Can you work these out from the model? Positions are in its coordinate system, mm. Face numbers are marked on the shaded views. Round coordinates to 2 decimals unless told otherwise and drop trailing zeros. Loops run counter-clockwise (first coordinate to the right, second up) from the corner with the lowest first, then second, coordinate; pieces in that order, holes last. Notation, with made-up numbers: M 0,64.25 L 27,64.25 A20 ccw 27,81.25 Z; hole C -31,37 d2. An arc over 180 degrees is marked long. Return JSON: item names as keys, results as strings.
```python
from build123d import *

# Parameters (mm, degrees)
BOSS_EXTRUDE1_DEPTH = 56.3
SKETCH2_R           = 8.37
CUT_EXTRUDE1_DEPTH  = 109.485473941


with BuildPart() as part:
    # Sketch1 → Boss-Extrude1 (new body)
    with BuildSketch(Plane(origin=(0, 0, 0), x_dir=(1, 0, 0), z_dir=(0, 1, 0))):
        with BuildLine():
            Line((-85.3, 58.95), (-87.3, 58.95))
            Line((-87.3, 58.95), (-87.3, 65.95))
            Line((-87.3, 65.95), (-82, 65.95))
            Line((-82, 65.95), (-57.085698874, 65.95))
            ThreePointArc((-57.085698874, 65.95), (-30.460620038, 81.733286627), (0, 87.224878997))
            ThreePointArc((0, 87.224878997), (30.460620038, 81.733286627), (57.085698874, 65.95))
            Line((57.085698874, 65.95), (82, 65.95))
            Line((82, 65.95), (87.3, 65.95))
            Line((87.3, 65.95), (87.3, 58.95))
            Line((87.3, 58.95), (85.3, 58.95))
            Line((85.3, 58.95), (85.3, 63.95))
            Line((85.3, 63.95), (82.7, 63.95))
            Line((82.7, 63.95), (82.7, 55.95))
            Line((82.7, 55.95), (77.3, 55.95))
            Line((77.3, 55.95), (77.3, 58.692745098))
            Line((77.3, 58.692745098), (78.85, 58.692745098))
            Line((78.85, 58.692745098), (79.85, 57.359411765))
            Line((79.85, 57.359411765), (81.3, 57.359411765))
            Line((81.3, 57.359411765), (81.3, 63.95))
            Line((81.3, 63.95), (56.335401836, 63.95))
            ThreePointArc((56.335401836, 63.95), (30.109375518, 79.728950237), (0, 85.224878997))
            ThreePointArc((0, 85.224878997), (-30.109375518, 79.728950237), (-56.335401836, 63.95))
            Line((-56.335401836, 63.95), (-81.3, 63.95))
            Line((-81.3, 63.95), (-81.3, 57.359411765))
            Line((-81.3, 57.359411765), (-79.85, 57.359411765))
            Line((-79.85, 57.359411765), (-78.85, 58.692745098))
            Line((-78.85, 58.692745098), (-77.3, 58.692745098))
            Line((-77.3, 58.692745098), (-77.3, 55.95))
            Line((-77.3, 55.95), (-82.7, 55.95))
            Line((-82.7, 55.95), (-82.7, 63.95))
            Line((-82.7, 63.95), (-85.3, 63.95))
            Line((-85.3, 63.95), (-85.3, 58.95))
        make_face()
    extrude(amount=BOSS_EXTRUDE1_DEPTH)

    # Sketch2 → Cut-Extrude1 (cut, through all)
    with BuildSketch(Plane.XY.offset(-55.95)):
        with Locations((12.955, 28.15)):
            Circle(SKETCH2_R)
        with Locations((-12.955, 28.15)):
            Circle(SKETCH2_R)
    extrude(amount=-CUT_EXTRUDE1_DEPTH, mode=Mode.SUBTRACT)


solid = part.part
```
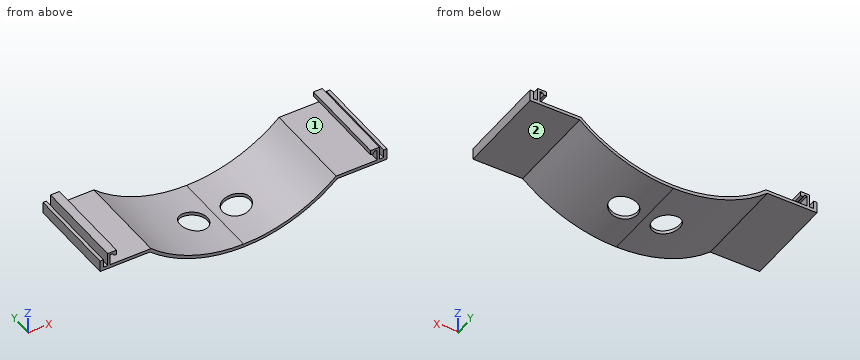
Q1. Suppose I cut it at A-A, the plane x = 17.5. Please give me the cut outline in (y, z), plus the area to 3 significant figures.
Results:
{"outline": "M 0,-85.45 L 21.12,-85.45 L 21.12,-83.41 L 0,-83.41 Z; M 35.18,-85.45 L 56.3,-85.45 L 56.3,-83.41 L 35.18,-83.41 Z", "area": "86.3 mm2"}
Q2. Thinking about a two-plate mould opening in X: for the marked faces 1 and 2, which applies, pulls with the +X half, pulls with the -X half, needs draft (parallel to the pull), parting line crosses it, or undercut?
Results:
{"face 1": "undercut", "face 2": "needs draft"}
Q3. If I drill on line 1 along X through (y, z) = (28.15, -85.4) (3 decimals); line 2 along Z through (x, y) = (58, 51); line 3 along X through (y, z) = (4.5, -79), over which ranges is the centre line in solid material (lowest first)?
Results:
{"line 1": "x = -4.585 to 4.585", "line 2": "z = -65.95 to -63.95", "line 3": "x = -36.98 to -31.97, 31.97 to 36.98"}
Q4. Suppose I cut it at C-C, the plane x = -60. Please give me the cut outline in (y, z), plus the area to 3 significant figures.
Results:
{"outline": "M 0,-65.95 L 56.3,-65.95 L 56.3,-63.95 L 0,-63.95 Z", "area": "113 mm2"}
Q5. Suppose I cut it at D-D, the plane y = 28.15. State how many separate pieces and enclosed holes the cut face has, plus the area to 3 significant figures.
Results:
{"separate pieces": "3", "enclosed holes": "0", "area": "361 mm2"}
Q6. I'm going to push flat-ended pins straight in: pin 1 Ø2 at (x, y) = (69.5, 45.5) entering from -Z; pin 2 Ø6 at (x, y) = (-51, 16.5) entering from -Z; pin 3 Ø4 at (x, y) = (36.5, 39) entering from +Z. Where does each tip first touch, or does it pass through?
Results:
{"pin 1": "stops at z = -65.95", "pin 2": "stops at z = -72.83", "pin 3": "stops at z = -76.03"}
Q7. Suppose I cut it at B-B, the plane y = 51. Please give me the cut outline in (x, z).
Results:
{"outline": "M -87.3,-65.95 L -57.09,-65.95 A87.22 ccw 57.09,-65.95 L 87.3,-65.95 L 87.3,-58.95 L 85.3,-58.95 L 85.3,-63.95 L 82.7,-63.95 L 82.7,-55.95 L 77.3,-55.95 L 77.3,-58.69 L 78.85,-58.69 L 79.85,-57.36 L 81.3,-57.36 L 81.3,-63.95 L 56.34,-63.95 A85.22 cw -56.34,-63.95 L -81.3,-63.95 L -81.3,-57.36 L -79.85,-57.36 L -78.85,-58.69 L -77.3,-58.69 L -77.3,-55.95 L -82.7,-55.95 L -82.7,-63.95 L -85.3,-63.95 L -85.3,-58.95 L -87.3,-58.95 Z"}
